CAD build for the part. Positions are in the model's coordinates, mm. A direction names the side the tool comes from. Coordinates: 2 decimals unless noted, no trailing zeros. Write each loop counter-clockwise with the first axis right and the second up, starting at its lowest first coordinate (ties: lowest second). Pieces come first, ordered by that corner, then holes. Notation, with made-up numbers: M 71,11.25 L 113,11.25 A17 ccw 113,26.25 Z; hole C 31.5,66.5 d9. An arc over 180 degrees is marked long. Put each result on its own line as item: value. Start each with the question number.
```python
from build123d import *

# Parameters (mm, degrees)
F0_R      = 22.355293723
F10_DEPTH = 25.4
F1_DEPTH  = 50.8
F11_DEPTH = 25.4
F3_DEPTH  = 25.4
F14_DEPTH = 25.4
F5_DEPTH  = 25.4
F6_R      = 9.2971028971
F7_DEPTH  = 76.201
F8_R      = 9.5875632129
F9_DEPTH  = 76.201


with BuildPart() as f10:
    # F0 (on Front) → F10 (new body)
    with BuildSketch(Plane.XZ):
        with Locations((0, -38.8152748346)):
            Circle(F0_R)
    extrude(amount=F10_DEPTH)

    # F1 (add): a face of the model
    f1_faces = [f10.faces().sort_by_distance(p)[0] for p in [
        (0, -25.4, -38.8152748346),
    ]]
    extrude(f1_faces, amount=F1_DEPTH)

    # F2 (on face) → F11 (join)
    with BuildSketch(Plane.XZ.offset(76.2)):
        with BuildLine():
            Line((18.6882317066, -26.5470576406), (18.6882317066, 50.6553947926))
            Line((18.6882317066, 50.6553947926), (-19.891411387, 50.6553947926))
            Line((-19.891411387, 50.6553947926), (-19.891411387, -28.6127795284))
            ThreePointArc((-19.891411387, -28.6127795284), (-1.1952874404, -16.4919586523), (18.6882317066, -26.5470576406))
        make_face()
    extrude(amount=-F11_DEPTH)

    # F12 (on face) → F3 (join)
    with BuildSketch(Plane(origin=(0, 0, 0), x_dir=(-1, 0, 0), z_dir=(0, 1, 0))):
        with BuildLine():
            Line((19.5738153324, 48.656180501), (-16.9442743063, 48.656180501))
            Line((-16.9442743063, 48.656180501), (-16.9442743063, -24.232726166))
            ThreePointArc((-16.9442743063, -24.232726166), (2.3036626211, -16.5789915128), (19.5738153324, -28.0159734325))
            Line((19.5738153324, -28.0159734325), (19.5738153324, 48.656180501))
        make_face()
    extrude(amount=-F3_DEPTH)

    # F13 (on face) → F14 (join)
    with BuildSketch(Plane.XZ.offset(76.2)):
        with BuildLine():
            Line((-19.891411387, 50.6553947926), (17.8490708054, 50.6553947926))
            ThreePointArc((17.8490708054, 50.6553947926), (-1.0211702908, 65.4485059403), (-19.891411387, 50.6553947926))
        make_face()
    extrude(amount=-F14_DEPTH)

    # F4 (on face) → F5 (join)
    with BuildSketch(Plane(origin=(0, 0, 0), x_dir=(-1, 0, 0), z_dir=(0, 1, 0))):
        with BuildLine():
            Line((-16.9442743063, 48.656180501), (18.7738145008, 48.656180501))
            ThreePointArc((18.7738145008, 48.656180501), (-4.1441192209, 66.9668983131), (-16.9442743063, 40.5723893641))
            Line((-16.9442743063, 40.5723893641), (-16.9442743063, 48.656180501))
        make_face()
    extrude(amount=-F5_DEPTH)

    # F6 (on face) → F7 (cut, through all)
    with BuildSketch(Plane.XZ.offset(76.2)):
        with Locations((0, 49.5857223868)):
            Circle(F6_R)
    extrude(amount=-F7_DEPTH, mode=Mode.SUBTRACT)

    # F8 (on face) → F9 (cut, through all)
    with BuildSketch(Plane.XZ.offset(76.2)):
        with Locations((0, -45.7826852798)):
            Circle(F8_R)
    extrude(amount=-F9_DEPTH, mode=Mode.SUBTRACT)


solid = f10.part
```
(1) Slice it at B-B, the plane z = 13.5. Write the cut outline in (x, y).
(2) Slice it at C-C, the plane y = -54. Write the cut outline in (x, z), then the cut area to 3 significant figures.
(3) Slice it at A-A, the plane x = 5. Write the cut outline in (y, z), then the cut area to 3 significant figures.
(4) Drill centre lines: line 1 (Z direction, x = 0, y = -61); line 2 (Z direction, x = 0, y = -23); line 3 (Z direction, x = 0, y = -44). Where is each one in solid material? Low to high. Write a range as [from, to].
(5) Drop flat-ended pins along their axis: pin 1 (6 mm diameter, centred on x = 11, y = -51.5, fed in from -Z); pin 2 (7.5 mm diameter, centred on y = -16, z = 12.5, fed in from -X); pin 3 (7.5 mm diameter, centred on y = -14, z = 16.5, fed in from +X); pin 4 (1.5 mm diameter, centred on x = 9, z = 33, fed in from +Y). Give the stop position or say it passes through.
(6) Which spindle directions (+Z, -Z, +X, -X, +Y, -Y) get a long thin tool onto all of the face, cutting with end or side? Do faces 4 (the face through (16.944, -13, 9)), 5 (the face through (-0.659, -63.678, 65.445)), 6 (the face through (-4.85, -37.57, -60.64)), 7 (the face through (-19.574, -13, 10)), 8 (the face through (-19.891, -64, 12)). Say none if no direction does.
(7) Two-plate mould, pull along X, no slides. Class faces 1 (the face through (-2.02, -63.68, 40.51)), 2 (the face through (18.688, -64, 12)), 3 (the face through (-1, -50.8, 19)): +X half, -X half, draft (parallel to the pull), parting line (faces both ways), or undercut.
(8) Slice it at D-D, the plane z = 56.5. Write the cut outline in (x, y).
Result set:
1. outline: M -19.89,-76.2 L 18.69,-76.2 L 18.69,-50.8 L -19.89,-50.8 Z; M -19.57,-25.4 L 16.94,-25.4 L 16.94,0 L -19.57,0 Z
2. outline: M -19.89,-28.61 A22.36 ccw long 18.69,-26.55 L 18.69,50.66 L 17.85,50.66 A19.43 ccw -19.89,50.66 Z; hole C 0,-45.78 d19.18; hole C 0,49.59 d18.59
2. area: 4,140 mm^2
3. outline: M -76.2,-60.6 L 0,-60.6 L 0,-53.96 L -76.2,-53.96 Z; M -76.2,-37.6 L 0,-37.6 L 0,41.75 L -25.4,41.75 L -25.4,-17.03 L -50.8,-17.03 L -50.8,41.75 L -76.2,41.75 Z; M -76.2,57.42 L -50.8,57.42 L -50.8,64.49 L -76.2,64.49 Z; M -25.4,57.42 L 0,57.42 L 0,66.75 L -25.4,66.75 Z
3. area: 5,480 mm^2
4. line 1: z = [-61.17, -55.37], [-36.2, 40.29], [58.88, 65.42]
4. line 2: z = [-61.17, -55.37], [-36.2, 40.29], [58.88, 67.43]
4. line 3: z = [-61.17, -55.37], [-36.2, -16.46]
5. pin 1: stops at z = -59.69
5. pin 2: stops at x = -19.57
5. pin 3: stops at x = 16.94
5. pin 4: stops at y = 0
6. face 4: +X, +Y
6. face 5: +Z, -Y
6. face 6: none
6. face 7: +Z, -X, +Y
6. face 8: +Z, -X, +Y, -Y
7. face 1: undercut
7. face 2: +X half
7. face 3: draft
8. outline: M -17.38,-76.2 L -6.22,-76.2 L -6.22,-50.8 L -17.38,-50.8 Z; M -17.06,-25.4 L -6.22,-25.4 L -6.22,0 L -17.06,0 Z; M 6.22,-76.2 L 15.34,-76.2 L 15.34,-50.8 L 6.22,-50.8 Z; M 6.22,-25.4 L 17.06,-25.4 L 17.06,0 L 6.22,0 Z
